Design review of the part built by this model. Coordinates are the model's own, in mm. A direction names the side the tool comes from. Coordinates: 2 decimals unless noted, no trailing zeros. Loops run counter-clockwise (first coordinate to the right, second up) from the corner with the lowest first, then second, coordinate; pieces in that order, holes last. Notation, with made-up numbers: M -37,71.25 L 11,71.25 A27 cw 11,91.25 Z; hole C 88.5,1 d5. An arc over 180 degrees is marked long. One line per item, written item: value.
Solid Edge part; units mm, degrees
sketch "Sketch1" plane through (0, 0, 0) normal (0, 0, 1) x (1, 0, 0)
  line L0 (-42.8211, -17.5263) -> (97.1789, -17.5263)
  line L1 (97.1789, -17.5263) -> (97.1789, 27.4737)
  line L2 (97.1789, 27.4737) -> (-42.8211, 27.4737)
  line L3 (-42.8211, 27.4737) -> (-42.8211, -17.5263)
extrude "Protrusion1" add sketch "Sketch1" along normal blind 12.5
hole "Hole_1" at (47.1789, 17.4737, 12.5) direction (0, 0, -1) diameter 11 end through all
hole "Hole1" at (7.1789, 17.4737, 12.5) direction (0, 0, -1) diameter 11 end through all
hole "Hole_3" at (79.6789, -3.0263, 12.5) direction (0, 0, -1) diameter 4.917 end through all
hole "Hole2" at (-25.3211, -0.0263, 12.5) direction (0, 0, -1) diameter 4.917 end through all
sketch "Sketch2" plane through (27.1789, 4.9737, 12.5) normal (0, 0, 1) x (1, 0, 0)
  line L0 (-38, -22.5) -> (-38, -3)
  arc A0 (-38, -3) -> (-33, 2) centre (-33, -3) cw
  line L1 (-33, 2) -> (33, 2)
  arc A1 (33, 2) -> (38, -3) centre (33, -3) cw
  line L2 (38, -3) -> (38, -22.5)
  line L3 (-38, -22.5) -> (38, -22.5)
  line L4 (25.5, 22.5) -> (70, 22.5)
  line L5 (70, 22.5) -> (70, 4.5)
  line L6 (70, 4.5) -> (25.5, 22.5)
  line L7 (-70, 22.5) -> (-25.5, 22.5)
  line L8 (-25.5, 22.5) -> (-70, 7.5)
  line L9 (-70, 7.5) -> (-70, 22.5)
extrude "Cutout1" cut sketch "Sketch2" against normal through all
sketch "Sketch3" plane through (27.1789, 4.9737, 12.5) normal (0, 0, 1) x (1, 0, 0)
  line L0 (-35, -19.5) -> (-35, -22.5)
  line L1 (-35, -22.5) -> (-75.0244, -22.5)
  line L2 (-75.0244, -22.5) -> (-75.0244, -19.5)
  line L3 (-75.0244, -19.5) -> (-35, -19.5)
  line L4 (70, -22.5) -> (67, -22.5)
  line L5 (67, -22.5) -> (67, 21.0516)
  line L6 (67, 21.0516) -> (70, 21.0516)
  line L7 (70, 21.0516) -> (70, -22.5)
  line L8 (-70, -22.5) -> (-67, -22.5)
  line L9 (-67, -22.5) -> (-67, 20.7963)
  line L10 (-67, 20.7963) -> (-70, 20.7963)
  line L11 (-70, 20.7963) -> (-70, -22.5)
extrude "Cutout2" cut sketch "Sketch3" against normal through all
sketch "Sketch4" plane through (27.1789, 4.9737, 12.5) normal (0, 0, 1) x (1, 0, 0)
  line L0 (-67, 7.5) -> (-25.5, 22.5)
  line L1 (-25.5, 22.5) -> (-67, 8.5112)
  line L2 (-67, 8.5112) -> (-67, 7.5)
extrude "Cutout3" cut sketch "Sketch4" against normal through all
properties material "Aluminum, 6061-T6"
(1) Tool access review of faces 5 (the cylindrical face through (-27.72, 0.51, 6.34)), 6 (the cylindrical face through (63.753, 5.47, 6.338)), 7 (the flat face through (-26, -14.526, 6)): name each direction out of +Z, -Z, +X, -X, +Y, -Y from which nothing blocks a thin tool from reaching the whole face with its end or side.
Reply:
face 5: +Z, -Z
face 6: +Z, -Z, -Y
face 7: +Z, -Z, -X, -Y
(2) Insertion check: pin 1 (2 mm diameter, centred on x = 12.5, z = 6, fed in from -Y); pin 2 (10 mm diameter, centred on x = 7.18, y = 17.47, fed in from +Z); pin 3 (2 mm diameter, centred on x = -12.5, z = 3, fed in from -Y). Each pin has a flat end and moves straight along its axis. Give the tip position at first contact, or say it passes through.
Reply:
pin 1: stops at y = 6.97
pin 2: passes through
pin 3: stops at y = -14.53
(3) We need section B-B on y = 19. State the section outline as (x, z) points (3 decimals).
Reply:
outline: M -21.765,0 L 1.895,0 L 1.895,12.5 L -21.765,12.5 Z; M 12.463,0 L 41.895,0 L 41.895,12.5 L 12.463,12.5 Z; M 52.463,0 L 73.628,0 L 73.628,12.5 L 52.463,12.5 Z
(4) We need section D-D on x = 24. State the section outline as (y, z) points.
Reply:
outline: M 6.97,0 L 27.47,0 L 27.47,12.5 L 6.97,12.5 Z
(5) To check wall thickness, follow line 1 along X through (y, z) = (0, 0.75); line 2 along X through (y, z) = (1.5, 5.75); line 3 along X through (y, z) = (-1.5, 11.5). State the ranges of each line that lie inside material, in increasing order. Write a range as [from, to].
Reply:
line 1: x = [-39.82, -27.78], [-22.86, -10.82], [65.18, 94.18]
line 2: x = [-39.82, -27.25], [-23.39, -10.82], [65.18, 94.18]
line 3: x = [-39.82, -27.29], [-23.35, -10.82], [65.18, 77.75], [81.61, 94.18]
(6) We need section A-A on y = -8.5. State the section outline as (x, z) points, then the cut area to 3 significant figures.
Reply:
outline: M -39.82,0 L -10.82,0 L -10.82,12.5 L -39.82,12.5 Z; M 65.18,0 L 94.18,0 L 94.18,12.5 L 65.18,12.5 Z
area: 725 mm2
(7) We need section C-C on z = 2. State the section outline as (x, y) points, then the cut area to 3 significant figures.
Reply:
outline: M -39.82,-14.53 L -10.82,-14.53 L -10.82,1.97 A5 cw -5.82,6.97 L 60.18,6.97 A5 cw 65.18,1.97 L 65.18,-17.53 L 94.18,-17.53 L 94.18,10.69 L 52.68,27.47 L 1.68,27.47 L -39.82,12.47 Z; hole C -25.32,-0.03 d4.92; hole C 7.18,17.47 d11; hole C 47.18,17.47 d11; hole C 79.68,-3.03 d4.92
area: 3,200 mm2
(8) Mouldability with a two-part tool opening along X and no side actions: class faces 1 (the flat face through (73.719, 18.963, 6.338)), 2 (the flat face through (28, 27.474, 6)), 3 (the flat face through (-10.821, -6, 6)), 4 (the flat face through (-39.821, -1, 6)) as released by +X, released by -X, zero draft, split by the parting line, or undercut.
Reply:
face 1: released by +X
face 2: zero draft
face 3: undercut
face 4: released by -X
